Read the model definition and answer for the solid it produces. Units are mm, in the model's axes. Round coordinates to 2 decimals unless told otherwise and drop trailing zeros. Write each loop counter-clockwise with the first axis right and the second up, starting at its lowest first coordinate (ties: lowest second). Pieces come first, ordered by that corner, then holes. Notation, with made-up numbers: M 59.25,50 L 84.25,50 A14 cw 84.25,67 Z; hole C 12.5,32.5 d9. An arc over 180 degrees is marked long. Use one line per item in the form item = value. Start each with the question number.
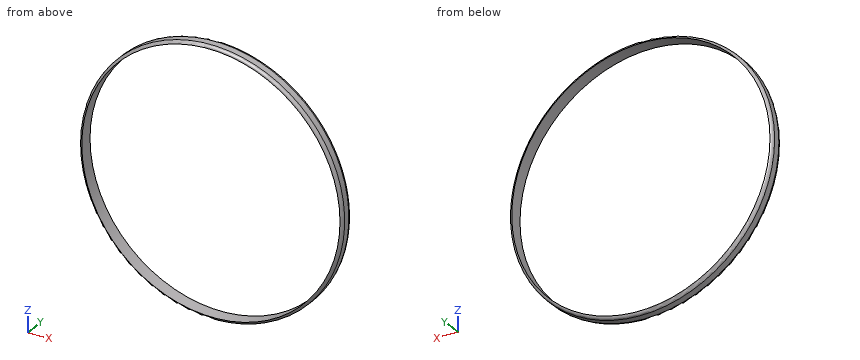
Autodesk Inventor part; units mm, degrees
ref_plane "YZ Plane" through (0, 0, 0) normal (1, 0, 0) x (0, 1, 0)
ref_plane "XZ Plane" through (0, 0, 0) normal (0, 1, 0) x (-1, 0, 0)
ref_plane "XY Plane" through (0, 0, 0) normal (0, 0, 1) x (1, 0, 0)
sketch "Sketch1" plane through (0, 0, 0) normal (0, 1, 0) x (-1, 0, 0)
  circle A0 centre (0, 0) radius 124.46
  circle A1 centre (0, 0) radius 127
  dimension "d0" = 248.92
  dimension "d1" = 254
extrude "Extrusion1" add sketch "Sketch1" along normal blind 12.7
fillet "Fillet1" radius 3.175 1 edges at (127, 12.7, 0)
fillet "Fillet2" radius 3.175 1 edges at (127, 0, 0)
properties part number "Prop_Ring"
Q1. Each of these flat-tipped pins is pushed along its axis until it touches: pin 1 Ø3 at (y, z) = (5.5, -6) entering from -X; pin 2 Ø1.5 at (y, z) = (4.5, 13.5) entering from +X; pin 3 Ø5 at (y, z) = (4.5, -19) entering from +X. Where does it stop, or does it pass through?
Q2. Find section B-B on z = 0. Write down the section's boundary in (x, y) (3 decimals).
Q3. Find section A-A on x = 0. Write down the section's boundary in (y, z) (3 decimals), and give its area (3 significant figures).
Q4. Find section C-C on y = 7. Write down the section's boundary in (x, z), and give its area (3 significant figures).
Q5. Straight lines are drawn through the part: line 1 (Z direction, x = 0, y = 9.75); line 2 (Z direction, x = -45.5, y = 4.25); line 3 (X direction, y = 2, z = -104). For each, find the intervals that lie inside material, in ascending order. Write a range as [from, to].
Response:
q1.pin_1 = -126.92
q1.pin_2 = 126.36
q1.pin_3 = 125.92
q2.outline = M -127,3.111 A3.175 ccw -124.46,0 L -124.46,12.7 A3.175 ccw -127,9.589 Z; M 124.46,0 A3.175 ccw 127,3.111 L 127,9.589 A3.175 ccw 124.46,12.7 Z
q3.outline = M 0,-124.46 A3.175 ccw 3.111,-127 L 9.589,-127 A3.175 ccw 12.7,-124.46 Z; M 0,124.46 L 12.7,124.46 A3.175 ccw 9.589,127 L 3.111,127 A3.175 ccw Z
q3.area = 56.6 mm²
q4.outline = C 0,0 d254; hole C 0,0 d248.92
q4.area = 2,010 mm²
q5.line_1 = [-127, -124.46], [124.46, 127]
q5.line_2 = [-118.57, -115.84], [115.84, 118.57]
q5.line_3 = [-72.54, -68.37], [68.37, 72.54]
